Answer from the drawing. Dimensions are ordinates in mm from the lowest x, y and z of the part. A direction names the side the tool comes from. Round coordinates to 2 decimals unless told otherwise and drop trailing zeros. Order: outer loops, then holes, each group sorted by start corner. A loop starts at its lowest first (then second) coordinate and runs counter-clockwise, first axis right, second up. Notation, with made-up numbers: M 40,13 L 70,13 A33 ccw 70,51 Z; hole C 48.5,-16 d10. An arc over 180 degrees is marked long. Write item = value, one per line. Start each with the question number.
(1) A cutting plane is placed at A-A, the plane x = 24. Determine the outline of the cut face in (y, z).
(2) For a pull along Z with two mould halves and no side action, classify the marked faces 1, 2, 3 and 4 as released by +Z, released by -Z, zero draft, split by the parting line, or undercut.
(3) Straight lines are drawn through the part: probe 1 along X at (y, z) = (26, 1.5); probe 2 along Y at (x, z) = (34.5, 1.5); probe 3 along X at (y, z) = (22, 2.5). For each, find the intervals that lie inside material, in ascending order. Write a range as from..to.
(4) Each of these flat-tipped pins is pushed along its axis until it touches: pin 1 (2.5 mm diameter, centred on x = 4.5, y = 15.86, fed in from +Z); pin 2 (4 mm diameter, centred on x = 48, z = 11, fed in from -Y). Where does it stop, or does it pass through?
(5) Which of the six approach directions +Z, -Z, +X, -X, +Y, -Y give full straight-line access (tool end or side, diameter ignored) to the marked faces 5 and 6?
(6) A cutting plane is placed at D-D, the plane z = 2.5. Determine the outline of the cut face in (x, y).
(7) A cutting plane is placed at C-C, the plane y = 29. Determine the outline of the cut face in (x, z), and give its area (3 significant figures).
(8) A cutting plane is placed at B-B, the plane y = 15.86. Determine the outline of the cut face in (x, z), and give its area (3 significant figures).
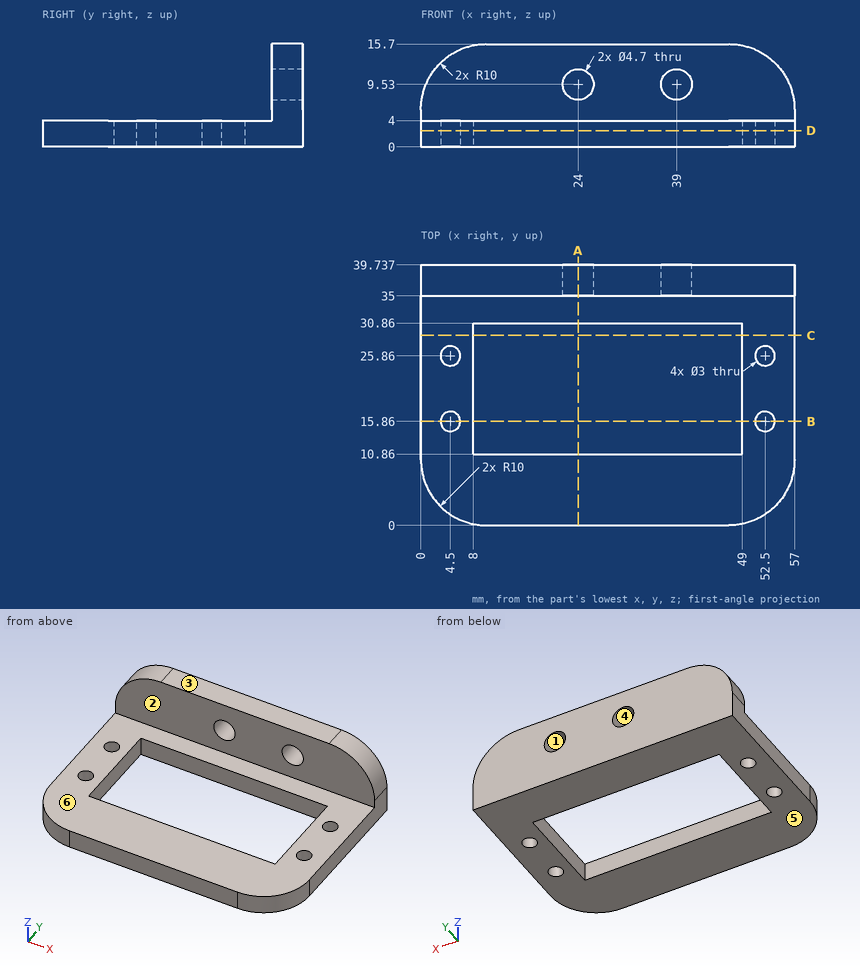
Reported:
q1.outline = M 0,0 L 10.86,0 L 10.86,4 L 0,4 Z; M 30.86,0 L 39.74,0 L 39.74,7.18 L 35,7.18 L 35,4 L 30.86,4 Z; M 35,11.88 L 39.74,11.88 L 39.74,15.7 L 35,15.7 Z
q2.face_1 = undercut
q2.face_2 = zero draft
q2.face_3 = released by +Z
q2.face_4 = undercut
q3.probe_1 = 0..3.01, 5.99..8, 49..51.01, 53.99..57
q3.probe_2 = 0..10.86, 30.86..39.74
q3.probe_3 = 0..8, 49..57
q4.pin_1 = through
q4.pin_2 = 35
q5.face_5 = -Z, +X, -X, +Y, -Y
q5.face_6 = +Z, +X, -X, -Y
q6.outline = M 0,10 A10 ccw 10,0 L 47,0 A10 ccw 57,10 L 57,39.74 L 0,39.74 Z; hole C 4.5,15.86 d3; hole C 4.5,25.86 d3; hole M 8,10.86 L 49,10.86 L 49,30.86 L 8,30.86 Z; hole C 52.5,15.86 d3; hole C 52.5,25.86 d3
q7.outline = M 0,0 L 8,0 L 8,4 L 0,4 Z; M 49,0 L 57,0 L 57,4 L 49,4 Z
q7.area = 64.0 mm²
q8.outline = M 0,0 L 3,0 L 3,4 L 0,4 Z; M 6,0 L 8,0 L 8,4 L 6,4 Z; M 49,0 L 51,0 L 51,4 L 49,4 Z; M 54,0 L 57,0 L 57,4 L 54,4 Z
q8.area = 40.0 mm²
